The listing builds one solid part. Answer for the finished solid, in the listing's coordinates (mm). A direction names the side the tool comes from. Coordinates: 2 decimals unless noted, no trailing zeros. Order: outer loops, then holes, each group sorted by start corner. A loop starts at its lowest first (then second) coordinate and runs counter-clockwise, first axis right, second up.
Autodesk Inventor part; units mm, degrees
ref_plane "YZ Plane" through (0, 0, 0) normal (1, 0, 0) x (0, 1, 0)
ref_plane "XZ Plane" through (0, 0, 0) normal (0, 1, 0) x (-1, 0, 0)
ref_plane "XY Plane" through (0, 0, 0) normal (0, 0, 1) x (1, 0, 0)
sketch "Sketch1" plane through (0, 0, 0) normal (0, 1, 0) x (-1, 0, 0)
  line L0 (19.05, 44.45) -> (-19.05, 44.45)
  line L1 (-19.05, 44.45) -> (-19.05, -44.45)
  line L2 (-19.05, -44.45) -> (19.05, -44.45)
  line L3 (19.05, -44.45) -> (19.05, 44.45)
  circle A0 centre (11.5, 29) radius 1.375 construction
  circle A1 centre (11.5, -29) radius 1.375 construction
  circle A2 centre (-11.5, 29) radius 1.375 construction
  circle A3 centre (-11.5, -29) radius 1.375 construction
  point P0 (0, 0)
  dimension "d0" = 88.9
  dimension "d1" = 38.1
  dimension "d2" = 19.05
  dimension "d3" = 44.45
  dimension "d4" = 2.75
  dimension "d5" = 2.75
  dimension "d6" = 2.75
  dimension "d7" = 2.75
  dimension "d8" = 58
  dimension "d9" = 58
  dimension "d10" = 23
  dimension "d11" = 11.5
  dimension "d12" = 29
  dimension "d13" = 29
  dimension "d14" = 23
  dimension "d15" = 11.5
extrude "Extrusion1" add sketch "Sketch1" along normal blind 3.175
sketch "Sketch2" plane through (0, 0, 0) normal (0, -1, 0) x (1, 0, 0)
  circle A0 centre (15.875, 41.275) radius 1.5875
  circle A1 centre (-15.875, 41.275) radius 1.5875
  circle A2 centre (-15.875, -41.275) radius 1.5875
  circle A3 centre (3.175, -41.275) radius 1.5875
  line L0 (-19.05, 44.45) -> (19.05, 44.45)
  line L1 (-19.05, -44.45) -> (-19.05, 44.45)
  line L2 (19.05, 44.45) -> (19.05, -44.45)
  line L3 (19.05, -44.45) -> (-19.05, -44.45)
  point P0 (0, 0)
  dimension "d18" = 3.175
  dimension "d19" = 3.175
  dimension "d20" = 3.175
  dimension "d21" = 3.175
  dimension "d22" = 15.875
  dimension "d23" = 3.175
  dimension "d24" = 3.175
  dimension "d25" = 3.175
  dimension "d26" = 3.175
  dimension "d27" = 3.175
  dimension "d28" = 3.175
  dimension "d29" = 3.175
extrude "Extrusion2" add sketch "Sketch2" along normal blind 18.415 contours A0 | A1 | A2 | A3
sketch "Sketch3" plane through (0, 3.175, 0) normal (0, 1, 0) x (1, 0, 0)
  circle A0 centre (-14.2875, 17.5562) radius 1.6764
  circle A1 centre (-14.2875, 31.75) radius 1.6764
  line L0 (19.05, -44.45) -> (19.05, 44.45)
  line L1 (-19.05, -44.45) -> (19.05, -44.45)
  line L2 (-14.2875, 31.75) -> (-14.2875, 17.5562) construction
  line L3 (-19.05, 44.45) -> (-19.05, -44.45)
  line L4 (19.05, 44.45) -> (-19.05, 44.45)
  point P0 (0, 0)
  dimension "d32" = 3.3528
  dimension "d33" = 3.3528
  dimension "d34" = 14.1938
  dimension "d39" = 4.7625
  dimension "d40" = 12.7
extrude "Extrusion3" [suppressed]
equation "\"d5\" = d4"
equation "\"d6\" = d4"
equation "\"d7\" = d4"
equation "\"d9\" = d8"
equation "\"d14\" = d10"
equation "\"d19\" = d18"
equation "\"d20\" = d21"
equation "\"d23\" = d18"
equation "\"d24\" = d18"
equation "\"d25\" = d21"
equation "\"d27\" = d26"
equation "\"d28\" = d26"
equation "\"d29\" = d26"
equation "\"d32\" = d33"
properties part number "Pi Holder Mk2" material "Aluminum 6061"
(1) Find section A-A on x = 16. Determine the outline of the cut face in (y, z) (3 decimals).
(2) Given pin 1 Ø5 at (y, z) = (-3, 1) entering from -X (3 decimals); pin 2 Ø2 at (x, z) = (-1, -13) entering from -Y, each flat-ended and moving along its own axis, determine where each tip first touches the part or whether it passes through.
(3) The mould has two halves that part along Z. Classify faces 3 (the cylindrical face through (2.831, -9.079, -39.725)), 4 (the cylindrical face through (-16.219, -9.079, -39.725)), 5 (the flat face through (3, -18.415, -41)): pulls with the +Z half, pulls with the -Z half, needs draft (parallel to the pull), parting line crosses it, or undercut.
(4) Find section B-B on y = -4.5. Determine the outline of the cut face in (x, z) (1 decimal).
(5) A tool of negligible diameter and unlimited length cuts with its end or side. For faces 1 (the flat face through (16, -18.415, 41)), 2 (the cylindrical face through (16.728, -9.079, 39.936)), from which of +Z, -Z, +X, -X, +Y, -Y can it reach the whole face along a straight path? Write none if from no direction.
(6) Find section C-C on z = 2.5. Determine the outline of the cut face in (x, y) (3 decimals).
(7) Find section D-D on x = 9.5. Determine the outline of the cut face in (y, z) (3 decimals).
(8) Find the intervals of material crossed by probe 1 along Y at (x, z) = (8.5, 12.5) (3 decimals); probe 2 along Z at (x, y) = (16, -4.5); probe 3 along Z at (x, y) = (-15.5, -11.75), in increasing order.
Resolved:
1. outline: (-18.415, 39.692) - (0, 39.692) - (0, -44.45) - (3.175, -44.45) - (3.175, 44.45) - (0, 44.45) - (0, 42.858) - (-18.415, 42.858) - close
2. pin 1: passes through
2. pin 2: stops at y = 0
3. face 3: parting line crosses it
3. face 4: undercut
3. face 5: needs draft
4. outline: circle Ø3.2 at (-15.9, -41.3); circle Ø3.2 at (-15.9, 41.3); circle Ø3.2 at (3.2, -41.3); circle Ø3.2 at (15.9, 41.3)
5. face 1: +Z, -Z, +X, -X, -Y
5. face 2: -Y
6. outline: (-19.05, 0) - (19.05, 0) - (19.05, 3.175) - (-19.05, 3.175) - close
7. outline: (0, -44.45) - (3.175, -44.45) - (3.175, 44.45) - (0, 44.45) - close
8. probe 1: y = 0 to 3.175
8. probe 2: z = 39.69 to 42.86
8. probe 3: z = -42.82 to -39.73, 39.73 to 42.82
